Input: part model. Units: mm. Frame: model coordinates. Coordinates: 2 decimals unless noted, no trailing zeros. Write each loop counter-clockwise with the first axis right and the second up, starting at its lowest first coordinate (ties: lowest second). Pieces come first, ordered by that corner, then holes. Notation, with made-up numbers: (79, 25) - (105, 25) arc R12 ccw to (105, 34) - close; hole circle Ø9 at (41, 78). An arc over 180 degrees is marked (long way). Use a Markdown table: item, result. Add a question column.
Q1. Section query C-C (y = 7.5). Return the cut outline in (x, z).
Q2. Section query B-B (x = 15). Return the cut outline in (y, z), then the cut area to 3 significant figures.
Q3. Material intervals for probe 1 along Z at (x, y) = (17.5, 15); probe 2 along X at (y, z) = (8, 52), sorted ascending. Write a range as from..to.
Q4. Section query A-A (z = -26.5). Return the cut outline in (x, y), then the cut area to 3 significant figures.
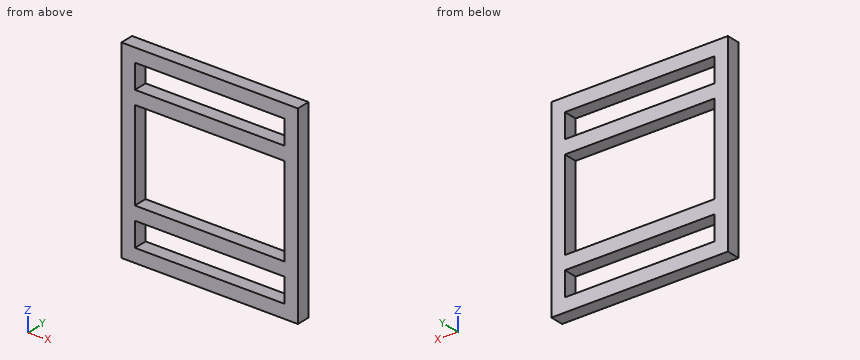
from build123d import *

# Parameters (mm, degrees)
SKETCH1_W           = 210
SKETCH1_H           = 34
SKETCH1_H_2         = 126
BOSS_EXTRUDE1_DEPTH = 19


with BuildPart() as part:
    # Sketch1 → Boss-Extrude1 (new body)
    with BuildSketch(Plane(origin=(0, 0, 0), x_dir=(1, 0, 0), z_dir=(0, 1, 0))):
        Polygon((-44.335030595, 191.764705882), (-44.335030595, -78.235294118), (-25.335030595, -78.235294118), (184.664969405, -78.235294118), (203.664969405, -78.235294118), (203.664969405, 191.764705882), (184.664969405, 191.764705882), (-25.335030595, 191.764705882), align=None)
        with Locations((79.664969405, -42.235294118)):
            Rectangle(SKETCH1_W, SKETCH1_H, mode=Mode.SUBTRACT)
        with Locations((79.664969405, 155.764705882)):
            Rectangle(SKETCH1_W, SKETCH1_H, mode=Mode.SUBTRACT)
        with Locations((79.664969405, 56.764705882)):
            Rectangle(SKETCH1_W, SKETCH1_H_2, mode=Mode.SUBTRACT)
    extrude(amount=BOSS_EXTRUDE1_DEPTH)


solid = part.part
Values follow:
| question | item | result |
|---|---|---|
| 1 | outline | (-44.34, -191.76) - (203.66, -191.76) - (203.66, 78.24) - (-44.34, 78.24) - close; hole (-25.34, -172.76) - (184.66, -172.76) - (184.66, -138.76) - (-25.34, -138.76) - close; hole (-25.34, -119.76) - (184.66, -119.76) - (184.66, 6.24) - (-25.34, 6.24) - close; hole (-25.34, 25.24) - (184.66, 25.24) - (184.66, 59.24) - (-25.34, 59.24) - close |
| 2 | outline | (0, -191.76) - (19, -191.76) - (19, -172.76) - (0, -172.76) - close; (0, -138.76) - (19, -138.76) - (19, -119.76) - (0, -119.76) - close; (0, 6.24) - (19, 6.24) - (19, 25.24) - (0, 25.24) - close; (0, 59.24) - (19, 59.24) - (19, 78.24) - (0, 78.24) - close |
| 2 | area | 1,440 mm2 |
| 3 | probe 1 | -191.76..-172.76, -138.76..-119.76, 6.24..25.24, 59.24..78.24 |
| 3 | probe 2 | -44.34..-25.34, 184.66..203.66 |
| 4 | outline | (-44.34, 0) - (-25.34, 0) - (-25.34, 19) - (-44.34, 19) - close; (184.66, 0) - (203.66, 0) - (203.66, 19) - (184.66, 19) - close |
| 4 | area | 722 mm2 |
